```python
from build123d import *

# Parameters (mm, degrees)
BOSS_EXTRUDE1_DEPTH = 6.35


with BuildPart() as part:
    # Model → Boss-Extrude1 (new body)
    with BuildSketch(Plane.XY):
        Polygon((1288.610132665, 22.860238699), (1300.745973293, 22.860238699), (1300.745973293, 28.575245224), (1312.176695005, 28.575245224), (1312.176695005, 22.860238699), (1323.607416717, 22.860238699), (1323.607416717, 28.575245224), (1335.038138429, 28.575245224), (1335.038138429, 22.860238699), (1346.46531683, 22.860238699), (1346.46531683, 28.575245224), (1357.896038543, 28.575245224), (1357.896038543, 22.860238699), (1369.326760255, 22.860238699), (1369.326760255, 28.575245224), (1380.757481967, 28.575245224), (1380.757481967, 22.860238699), (1392.188203679, 22.860238699), (1392.188203679, 28.575245224), (1403.615382081, 28.575245224), (1403.615382081, 22.860238699), (1415.046103793, 22.860238699), (1415.046103793, 28.575245224), (1426.476825505, 28.575245224), (1426.476825505, 22.860238699), (1437.907547217, 22.860238699), (1437.907547217, 28.575245224), (1449.33826893, 28.575245224), (1449.33826893, 22.860238699), (1461.470566246, 22.860238699), (1461.470566246, 28.575245224), (1461.470566246, 51.435413056), (1461.081244935, 54.393369189), (1459.939855837, 57.150419581), (1458.123908882, 59.517571103), (1455.75520539, 61.334361366), (1453.389602295, 63.150485487), (1451.574098254, 65.517240157), (1450.429608758, 68.274290549), (1450.039844534, 71.232246682), (1450.039844534, 245.918194159), (1450.429608758, 248.876284937), (1451.574098254, 251.633200684), (1453.389602295, 254.00013252), (1455.75520539, 255.816433806), (1458.123908882, 257.633089424), (1459.939855837, 260.000375591), (1461.081244935, 262.757291337), (1461.470566246, 265.715382116), (1461.470566246, 288.575408216), (1461.470566246, 294.290414741), (1449.33826893, 294.290414741), (1449.33826893, 288.575408216), (1437.907547217, 288.575408216), (1437.907547217, 294.290414741), (1426.476825505, 294.290414741), (1426.476825505, 288.575408216), (1415.046103793, 288.575408216), (1415.046103793, 294.290414741), (1403.615382081, 294.290414741), (1403.615382081, 288.575408216), (1392.188203679, 288.575408216), (1392.188203679, 294.290414741), (1380.757481967, 294.290414741), (1380.757481967, 288.575408216), (1369.326760255, 288.575408216), (1369.326760255, 294.290414741), (1357.896038543, 294.290414741), (1357.896038543, 288.575408216), (1346.46531683, 288.575408216), (1346.46531683, 294.290414741), (1335.038138429, 294.290414741), (1335.038138429, 288.575408216), (1323.607416717, 288.575408216), (1323.607416717, 294.290414741), (1312.176695005, 294.290414741), (1312.176695005, 288.575408216), (1300.745973293, 288.575408216), (1300.745973293, 294.290414741), (1288.610132665, 294.290414741), (1288.610132665, 288.575408216), (1288.610132665, 28.575245224), align=None)
        Polygon((1444.328026989, 44.27508992), (1444.328026989, 38.560083395), (1438.612666133, 38.560083395), (1438.612666133, 49.990096445), (1444.328026989, 49.990096445), align=None, mode=Mode.SUBTRACT)
        Polygon((1444.328026989, 67.13511602), (1444.328026989, 61.420109495), (1438.612666133, 61.420109495), (1438.612666133, 72.850122545), (1444.328026989, 72.850122545), align=None, mode=Mode.SUBTRACT)
        Polygon((1444.328026989, 89.99514212), (1444.328026989, 84.280135595), (1438.612666133, 84.280135595), (1438.612666133, 95.710148645), (1444.328026989, 95.710148645), align=None, mode=Mode.SUBTRACT)
        Polygon((1444.328026989, 112.85516822), (1444.328026989, 107.140161695), (1438.612666133, 107.140161695), (1438.612666133, 118.570174745), (1444.328026989, 118.570174745), align=None, mode=Mode.SUBTRACT)
        Polygon((1444.328026989, 135.71519432), (1444.328026989, 130.000187795), (1438.612666133, 130.000187795), (1438.612666133, 141.430200846), (1444.328026989, 141.430200846), align=None, mode=Mode.SUBTRACT)
        Polygon((1444.328026989, 158.575220421), (1444.328026989, 152.860213896), (1438.612666133, 152.860213896), (1438.612666133, 164.290226946), (1444.328026989, 164.290226946), align=None, mode=Mode.SUBTRACT)
        Polygon((1444.328026989, 181.435246521), (1444.328026989, 175.720239996), (1438.612666133, 175.720239996), (1438.612666133, 187.150253046), (1444.328026989, 187.150253046), align=None, mode=Mode.SUBTRACT)
        Polygon((1444.328026989, 204.295272621), (1444.328026989, 198.580266096), (1438.612666133, 198.580266096), (1438.612666133, 210.010279146), (1444.328026989, 210.010279146), align=None, mode=Mode.SUBTRACT)
        Polygon((1444.328026989, 227.155298721), (1444.328026989, 221.440292196), (1438.612666133, 221.440292196), (1438.612666133, 232.870305246), (1444.328026989, 232.870305246), align=None, mode=Mode.SUBTRACT)
        Polygon((1444.328026989, 250.015324821), (1444.328026989, 244.300318296), (1438.612666133, 244.300318296), (1438.612666133, 255.730331346), (1444.328026989, 255.730331346), align=None, mode=Mode.SUBTRACT)
        Polygon((1444.328026989, 272.875350921), (1444.328026989, 267.160344396), (1438.612666133, 267.160344396), (1438.612666133, 278.590357446), (1444.328026989, 278.590357446), align=None, mode=Mode.SUBTRACT)
    extrude(amount=BOSS_EXTRUDE1_DEPTH)


solid = part.part
```
Check sheet for the modelled part. Datum: model origin and axes. Units: mm. A direction names the side the tool comes from. Coordinates: 2 decimals unless noted, no trailing zeros. Write each loop counter-clockwise with the first axis right and the second up, starting at its lowest first coordinate (ties: lowest second). Pieces come first, ordered by that corner, then holes. Notation, with made-up numbers: (70.5, 43.25) -> (121.5, 43.25) arc R28 cw to (121.5, 62.25) -> close; hole circle Ø1 at (82.25, 71). An arc over 180 degrees is marked (long way). Use a Markdown table: item, result.
1. Scan lines: line 1 along X through (y, z) = (228, 4); line 2 along X through (y, z) = (275.5, 1.25); line 3 along X through (y, z) = (175.5, 5.25). Record each from-to range of solid material in increasing order.
Reported:
| item | result |
|---|---|
| line 1 | x = 1288.61 to 1438.61, 1444.33 to 1450.04 |
| line 2 | x = 1288.61 to 1438.61, 1444.33 to 1461.47 |
| line 3 | x = 1288.61 to 1450.04 |
2. Sectioned sample at B-B (z = 5). Give the number of separate pieces and of enclosed holes in the cut face, plus the area to 3 significant figures.
Reported:
| item | result |
|---|---|
| separate pieces | 1 |
| enclosed holes | 11 |
| area | 43,100 mm2 |
3. Release check for a two-part mould opening along Y. For faces 1 (the flat face through (1437.908, 291, 3)), 2 (the flat face through (1444, 288.575, 3)), 3 (the flat face through (1444.328, 113, 3)), 4 (the flat face through (1441, 118.57, 3)) record: pulls with the +Y half, pulls with the -Y half, needs draft (parallel to the pull), parting line crosses it, or undercut.
Reported:
| item | result |
|---|---|
| face 1 | needs draft |
| face 2 | pulls with the +Y half |
| face 3 | undercut |
| face 4 | undercut |
4. Sectioned sample at C-C (y = 101). Enter the section's corners in (x, z), plus the area to 3 significant figures.
Reported:
| item | result |
|---|---|
| outline | (1288.61, 0) -> (1450.04, 0) -> (1450.04, 6.35) -> (1288.61, 6.35) -> close |
| area | 1,030 mm2 |
5. Sectioned sample at A-A (y = 138.5). Enter the section's corners in (x, z).
Reported:
| item | result |
|---|---|
| outline | (1288.61, 0) -> (1438.61, 0) -> (1438.61, 6.35) -> (1288.61, 6.35) -> close; (1444.33, 0) -> (1450.04, 0) -> (1450.04, 6.35) -> (1444.33, 6.35) -> close |
6. Tool access check on faces 5 (the flat face through (1438.613, 136, 3)), 6 (the flat face through (1461.471, 280, 3)), 7 (the flat face through (1392.188, 291, 3)), 8 (the flat face through (1432, 294.29, 3)), 9 (the flat face through (1352, 28.575, 3)). Record the directions out of +Z, -Z, +X, -X, +Y, -Y that give a thin tool (end or side, any length) a straight path to the whole face; none if there is none.
Reported:
| item | result |
|---|---|
| face 5 | +Z, -Z |
| face 6 | +Z, -Z, +X, +Y, -Y |
| face 7 | +Z, -Z, +Y |
| face 8 | +Z, -Z, +X, -X, +Y |
| face 9 | +Z, -Z, -Y |
7. Go/stop test with flat-tipped pins: pin 1 Ø1.7 at (x, z) = (1440.5, 2) entering from +Y; pin 2 Ø1.5 at (y, z) = (227.5, 3) entering from +X; pin 3 Ø3 at (x, z) = (1445, 4.5) entering from -Y. Record where each tip stops, or that it passes through.
Reported:
| item | result |
|---|---|
| pin 1 | stops at y = 288.58 |
| pin 2 | stops at x = 1450.04 |
| pin 3 | stops at y = 28.58 |
8. Sectioned sample at D-D (x = 1422.5). Enter the section's corners in (y, z).
Reported:
| item | result |
|---|---|
| outline | (28.58, 0) -> (288.58, 0) -> (288.58, 6.35) -> (28.58, 6.35) -> close |
